Autodesk Inventor part; units mm, degrees
ref_plane "YZ Plane" through (0, 0, 0) normal (1, 0, 0) x (0, 1, 0)
ref_plane "XZ Plane" through (0, 0, 0) normal (0, 1, 0) x (-1, 0, 0)
ref_plane "XY Plane" through (0, 0, 0) normal (0, 0, 1) x (1, 0, 0)
sketch "Sketch1" plane through (0, 0, 0) normal (1, 0, 0) x (0, 1, 0)
  line L0 (20, 20) -> (-20, 20)
  arc A0 (5.6, -19.2) -> (-5.6, -19.2) centre (0, -15) ccw
  line L1 (-20, 20) -> (20, 20)
  arc A1 (19.2, 5.6) -> (19.2, -5.6) centre (15, 0) ccw
  line L2 (-20, 20) -> (20, 20)
  arc A2 (-19.2, -5.6) -> (-19.2, 5.6) centre (-15, 0) ccw
  line L3 (20, 20) -> (-20, 20)
  line L4 (-20, -20) -> (-6, -20)
  line L5 (6, -20) -> (20, -20)
  line L6 (-20, 20) -> (-20, 6)
  line L7 (-20, -6) -> (-20, -20)
  line L8 (20, -20) -> (20, -6)
  line L9 (20, 6) -> (20, 20)
  line L10 (20, 20) -> (20, 6)
  line L11 (20, -6) -> (20, -20)
  line L12 (-20, -20) -> (-20, -6)
  line L13 (-20, 6) -> (-20, 20)
  arc A3 (19.2, 5.6) -> (20, 6) centre (19.5, 6) ccw
  arc A4 (20, -6) -> (19.2, -5.6) centre (19.5, -6) ccw
  arc A5 (-6, -20) -> (-5.6, -19.2) centre (-6, -19.5) ccw
  arc A6 (5.6, -19.2) -> (6, -20) centre (6, -19.5) ccw
  arc A7 (-19.2, -5.6) -> (-20, -6) centre (-19.5, -6) ccw
  arc A8 (-20, 6) -> (-19.2, 5.6) centre (-19.5, 6) ccw
  point P0 (0, 0)
  point P1 (-4.899, -20)
  point P2 (4.899, -20)
  dimension "d3" = 40
  dimension "d4" = 40
  dimension "d5" = 40
  dimension "d9" = 14
  dimension "d10" = 0.5
  dimension "d11" = 0.5
extrude "Extrusion1" add sketch "Sketch1" along normal mid plane 2000
properties part number "launchrail"
Check sheet for the modelled part. Datum: model origin and axes. Units: mm. Give positions to 0.01 mm unless a question says otherwise; leave off trailing zeros. Order: outer loops, then holes, each group sorted by start corner. A loop starts at its lowest first (then second) coordinate and runs counter-clockwise, first axis right, second up. Notation, with made-up numbers: M -11.75,68.5 L 46.25,68.5 A20 cw 46.25,100.5 Z; hole C -35.75,80.25 d7. An arc over 180 degrees is marked long. Answer as CSV lines item,"result". Start each with the question number.
Item 1: Gauge pin test, flat ends, axial feed: P1, Ø3, axis at x = -693, z = -2.5, coming from the -Y side; P2, Ø8.5, axis at y = 0, z = -15, coming from the -X side. Record the tip position at first contact, or that the pin passes through.
Item 2: Thickness scan on line 1 (Y direction, x = -409.5, z = -15); line 2 (Z direction, x = 550, y = 13). Record the ranges inside material, lowest first. Write a range as [from, to].
Item 3: Cross-section at A-A on x = -372.5. Enter the section's corners in (y, z), plus the area to 3 significant figures.
Established:
1,P1,"stops at y = -9.26"
1,P2,"passes through"
2,line 1,"y = [-20, -7], [7, 20]"
2,line 2,"z = [-20, -6.71], [6.71, 20]"
3,outline,"M -20,-20 L -6,-20 A0.5 ccw -5.6,-19.2 A7 cw long 5.6,-19.2 A0.5 ccw 6,-20 L 20,-20 L 20,-6 A0.5 ccw 19.2,-5.6 A7 cw long 19.2,5.6 A0.5 ccw 20,6 L 20,20 L -20,20 L -20,6 A0.5 ccw -19.2,5.6 A7 cw long -19.2,-5.6 A0.5 ccw -20,-6 Z"
3,area,"1,180 mm^2"
